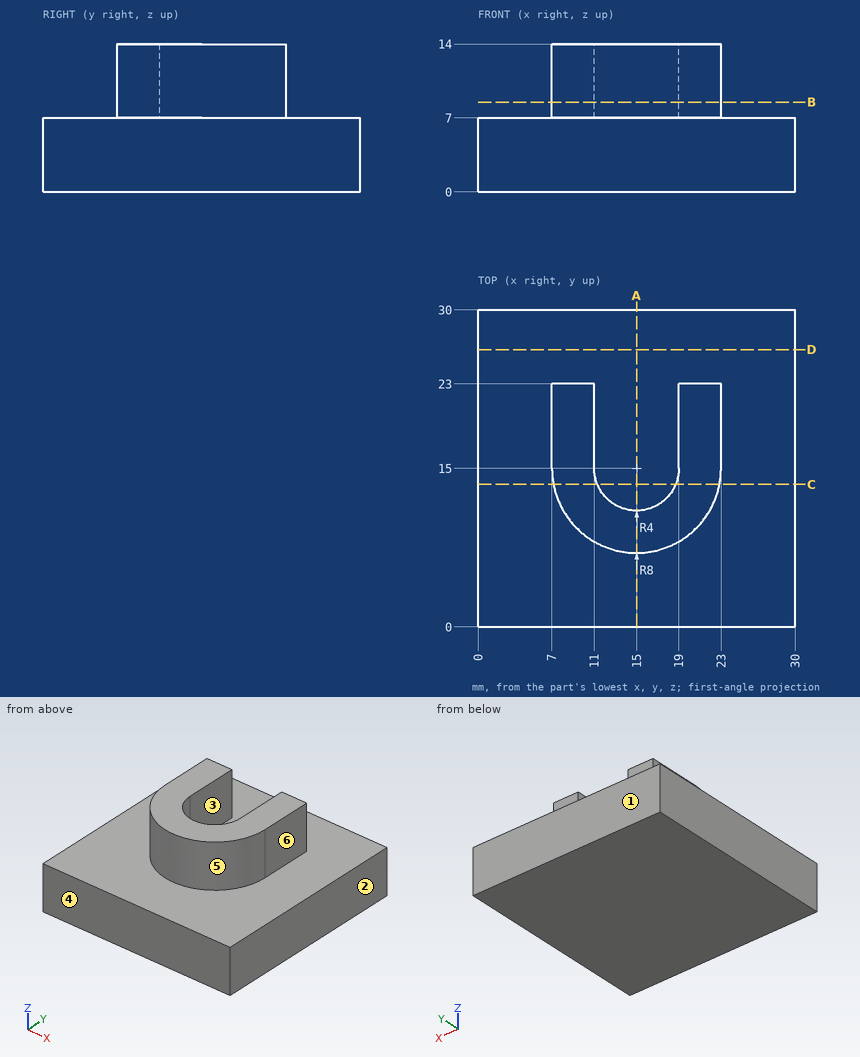
Can you work these out from the drawing? Everything is in mm from the part's minimum corner. A direction names the side the tool comes from. Give positions to 0.01 mm unless a question says otherwise; leave off trailing zeros. Order: outer loops, then holes, each group sorted by start corner. A loop starts at its lowest first (then second) coordinate and runs counter-clockwise, first axis right, second up. Notation, with made-up numbers: M 58.25,-0.75 L 75.25,-0.75 A11 ccw 75.25,17.25 Z; hole C 73,-17 d1. An arc over 180 degrees is marked long. Use a Markdown table: item, result. Add a question column.
1. Suppose I cut it at A-A (x = 15). List the corners of the cut face in (y, z) for me, and give its area (3 significant figures).
2. For pin 1 Ø2 at (x, z) = (9, 10) entering from +Y; pin 2 Ø1 at (x, y) = (15, 15.5) entering from +Z; pin 3 Ø12 at (x, y) = (24, 13.5) entering from -Z; pin 4 Ø3.5 at (y, z) = (20.5, 10) entering from +X, each with a flat end and sliding along its axis, tell me the tip position at first contact or that it passes through.
3. Suppose I cut it at B-B (z = 8.5). List the corners of the cut face in (x, y) for me.
4. If we mould it in two halves opening along X, with no side actions, what happens to the marked faces 1, 2 and 3? For each: +X half, -X half, draft (parallel to the pull), parting line (faces both ways), or undercut.
5. I need wall thicknesses on probe 1 along X at (y, z) = (17.75, 10.5); probe 2 along Z at (x, y) = (28.75, 12); probe 3 along X at (y, z) = (12.75, 12.5). Which ranges of each line are inside material? Lowest first, please. Write a range as from..to.
6. Suppose I cut it at C-C (y = 13.5). List the corners of the cut face in (x, z) for me.
7. On a 3-axis mill with a long thin cutter (end or side, diameter ignored), from which of +Z, -Z, +X, -X, +Y, -Y can I reach the whole of each face in a straight line? I mean the marked faces 4, 5 and 6. Say none if no direction works.
8. Suppose I cut it at D-D (y = 26.25). List the corners of the cut face in (x, z) for me.
Results list:
| question | item | result |
|---|---|---|
| 1 | outline | M 0,0 L 30,0 L 30,7 L 11,7 L 11,14 L 7,14 L 7,7 L 0,7 Z |
| 1 | area | 238 mm² |
| 2 | pin 1 | stops at y = 23 |
| 2 | pin 2 | stops at z = 7 |
| 2 | pin 3 | stops at z = 0 |
| 2 | pin 4 | stops at x = 23 |
| 3 | outline | M 7,15 A8 ccw 23,15 L 23,23 L 19,23 L 19,15 A4 cw 11,15 L 11,23 L 7,23 Z |
| 4 | face 1 | draft |
| 4 | face 2 | +X half |
| 4 | face 3 | undercut |
| 5 | probe 1 | x = 7..11, 19..23 |
| 5 | probe 2 | z = 0..7 |
| 5 | probe 3 | x = 7.32..11.69, 18.31..22.68 |
| 6 | outline | M 0,0 L 30,0 L 30,7 L 22.86,7 L 22.86,14 L 18.71,14 L 18.71,7 L 11.29,7 L 11.29,14 L 7.14,14 L 7.14,7 L 0,7 Z |
| 7 | face 4 | +Z, -Z, +X, -X, -Y |
| 7 | face 5 | +Z, -Y |
| 7 | face 6 | +Z, +X, +Y, -Y |
| 8 | outline | M 0,0 L 30,0 L 30,7 L 0,7 Z |
